from build123d import *

# Parameters (mm, degrees)
F0_W      = 609.6
F0_H      = 1079.5
F1_DEPTH  = 25.4
F2_W      = 609.6
F2_H      = 12.7
F3_DEPTH  = 609.6
F4_W      = 609.6
F4_H      = 12.7
F5_DEPTH  = 609.6
F6_W      = 609.6
F6_H      = 12.7
F7_DEPTH  = 609.6
F8_W      = 609.6
F8_H      = 12.7
F9_DEPTH  = 609.6
F10_W     = 609.6
F10_H     = 12.7
F11_DEPTH = 609.6
F13_R     = 5.08
F14_R     = 5.08
F15_R     = 5.08
F16_R     = 5.08
F17_R     = 5.08
F18_R     = 5.08


with BuildPart() as f1:
    # F0 (on Right) → F1 (new body)
    with BuildSketch(Plane.YZ):
        with Locations((304.8, 539.75)):
            Rectangle(F0_W, F0_H)
    extrude(amount=F1_DEPTH)

    # F2 (on face) → F3 (join)
    with BuildSketch(Plane.YZ.offset(25.4)):
        with Locations((304.8, 6.35)):
            Rectangle(F2_W, F2_H)
    extrude(amount=F3_DEPTH)

    # F4 (on face) → F5 (join)
    with BuildSketch(Plane.YZ.offset(25.4)):
        with Locations((304.8, 349.25)):
            Rectangle(F4_W, F4_H)
    extrude(amount=F5_DEPTH)

    # F6 (on face) → F7 (join)
    with BuildSketch(Plane.YZ.offset(25.4)):
        with Locations((304.8, 692.15)):
            Rectangle(F6_W, F6_H)
    extrude(amount=F7_DEPTH)

    # F8 (on face) → F9 (join)
    with BuildSketch(Plane.YZ.offset(25.4)):
        with Locations((304.8, 882.65)):
            Rectangle(F8_W, F8_H)
    extrude(amount=F9_DEPTH)

    # F10 (on face) → F11 (join)
    with BuildSketch(Plane.YZ.offset(25.4)):
        with Locations((304.8, 1073.15)):
            Rectangle(F10_W, F10_H)
    extrude(amount=F11_DEPTH)

    # F12: F1 across face


with BuildPart() as f1_1:
    add(f1.part)
    add(f1.part.mirror(Plane(origin=(635, 304.8, 6.35), x_dir=(0, 1, 0), z_dir=(1, 0, 0))))

    # F13
    f13_edges = [f1_1.edges().sort_by_distance(p)[0] for p in [
        (0, 304.8, 1079.5),
    ]]
    fillet(f13_edges, radius=F13_R)

    # F14
    f14_edges = [f1_1.edges().sort_by_distance(p)[0] for p in [
        (1270, 304.8, 1079.5),
    ]]
    fillet(f14_edges, radius=F14_R)

    # F15
    f15_edges = [f1_1.edges().sort_by_distance(p)[0] for p in [
        (1270, 304.8, 0),
    ]]
    fillet(f15_edges, radius=F15_R)

    # F16
    f16_edges = [f1_1.edges().sort_by_distance(p)[0] for p in [
        (0, 304.8, 0),
    ]]
    fillet(f16_edges, radius=F16_R)

    # F17
    f17_edges = [f1_1.edges().sort_by_distance(p)[0] for p in [
        (635, 0, 1079.5),
    ]]
    fillet(f17_edges, radius=F17_R)

    # F18
    f18_edges = [f1_1.edges().sort_by_distance(p)[0] for p in [
        (635, 609.6, 1079.5),
    ]]
    fillet(f18_edges, radius=F18_R)


solid = f1_1.part
Build history of the part. All positions in model axes, mm. A direction names the side the tool comes from. Round coordinates to 2 decimals unless told otherwise and drop trailing zeros. Write each loop counter-clockwise with the first axis right and the second up, starting at its lowest first coordinate (ties: lowest second). Pieces come first, ordered by that corner, then holes. Notation, with made-up numbers: (32.25, 42.5) - (66.25, 42.5) arc R31 cw to (66.25, 73.5) - close; hole circle Ø7 at (72, 56). An arc over 180 degrees is marked (long way). One line per question, with ' | ' between items.
1. Drill centre lines: line 1 along Z through (x, y) = (489, 496.5); line 2 along X through (y, z) = (166.5, 271). Where is each one in solid material? Low to high. Write a range as from..to.
Results are:
line 1: 0..12.7, 342.9..355.6, 685.8..698.5, 876.3..889, 1066.8..1079.5 | line 2: 0..25.4, 1244.6..1270
2. Band-saw the part on B-B, the plane z = 666.5. Write the cut outline in (x, y).
Results are:
outline: (0, 5.08) arc R5.08 ccw to (5.08, 0) - (25.4, 0) - (25.4, 609.6) - (5.08, 609.6) arc R5.08 ccw to (0, 604.52) - close; (1244.6, 0) - (1264.92, 0) arc R5.08 ccw to (1270, 5.08) - (1270, 604.52) arc R5.08 ccw to (1264.92, 609.6) - (1244.6, 609.6) - close
3. Mould opens along Z. For faces 3 (the face through (644, 301, 0)), 4 (the face through (644, 301, 876.3)), 5 (the face through (638, 0, 696)) say: released by +Z, released by -Z, zero draft, split by the parting line, or undercut.
Results are:
face 3: released by -Z | face 4: undercut | face 5: zero draft
4. Band-saw the part on A-A, the plane x = 555.5. Write the cut outline in (y, z), and give its area (3 significant figures).
Results are:
outline: (0, 5.08) arc R5.08 ccw to (5.08, 0) - (604.52, 0) arc R5.08 ccw to (609.6, 5.08) - (609.6, 12.7) - (0, 12.7) - close; (0, 342.9) - (609.6, 342.9) - (609.6, 355.6) - (0, 355.6) - close; (0, 685.8) - (609.6, 685.8) - (609.6, 698.5) - (0, 698.5) - close; (0, 876.3) - (609.6, 876.3) - (609.6, 889) - (0, 889) - close; (0, 1066.8) - (609.6, 1066.8) - (609.6, 1074.42) arc R5.08 ccw to (604.52, 1079.5) - (5.08, 1079.5) arc R5.08 ccw to (0, 1074.42) - close | area: 38,700 mm^2
5. Tool access for faces 1 (the face through (644, 301, 698.5)), 2 (the face through (644, 301, 1079.5)): list every direction of +Z, -Z, +X, -X, +Y, -Y with a clear straight run to the whole face (end or side of a thin tool).
Results are:
face 1: +Y, -Y | face 2: +Z, +X, -X, +Y, -Y
6. Band-saw the part on C-C, the plane y = 88. Write the cut outline in (x, z), and give its area (3 significant figures).
Results are:
outline: (0, 5.08) arc R5.08 ccw to (5.08, 0) - (1264.92, 0) arc R5.08 ccw to (1270, 5.08) - (1270, 1074.42) arc R5.08 ccw to (1264.92, 1079.5) - (5.08, 1079.5) arc R5.08 ccw to (0, 1074.42) - close; hole (25.4, 12.7) - (1244.6, 12.7) - (1244.6, 342.9) - (25.4, 342.9) - close; hole (25.4, 355.6) - (1244.6, 355.6) - (1244.6, 685.8) - (25.4, 685.8) - close; hole (25.4, 698.5) - (1244.6, 698.5) - (1244.6, 876.3) - (25.4, 876.3) - close; hole (25.4, 889) - (1244.6, 889) - (1244.6, 1066.8) - (25.4, 1066.8) - close | area: 132,000 mm^2
